The listing builds one solid part. Answer for the finished solid, in the listing's coordinates (mm). A direction names the side the tool comes from. Coordinates: 2 decimals unless noted, no trailing zeros. Order: outer loops, then holes, each group sorted by start corner. A loop starts at its lowest first (then second) coordinate and runs counter-clockwise, first axis right, second up. Notation, with made-up numbers: (83.5, -36.75) -> (99.5, -36.75) arc R13 cw to (99.5, -20.75) -> close; hole circle Ø4 at (9, 10). An arc over 180 degrees is marked (long way). Write each question's results on one line, items separated by ' | '. Start each with the question number.
(1) The part is cut by section B-B, the plane y = 13.25. Give the vertices of the cut face in (x, z).
(2) Straight lines are drawn through the part: L1, parallel to Y at x = 40, z = -40.5; L2, parallel to Z at x = -40.5, y = 14.5; L3, parallel to Z at x = -23.5, y = 1.5. For each, find the intervals that lie inside material, in ascending order.
(3) Determine the mould class of faces 3 (the face through (-50, 23, 24)), 4 (the face through (-53.3, 1, 14.7)), 5 (the face through (-0.195, -0.521, 61.487)), 6 (the face through (-62, 10.37, -19.52)) for opening direction Y: +Y half, -Y half, draft (parallel to the pull), parting line (faces both ways), or undercut.
(4) A tool of negligible diameter and unlimited length cuts with its end or side. For faces 1 (the face through (-53.3, 20, -14.7)), 2 (the face through (-0.195, 21.479, 61.487)), from which of +Z, -Z, +X, -X, +Y, -Y can it reach the whole face along a straight path? Write none if from no direction.
(5) The part is cut by section A-A, the plane z = -10. Give the vertices of the cut face in (x, y), then the cut area to 3 significant figures.
(6) The part is cut by section C-C, the plane x = -7.5. Give the vertices of the cut face in (y, z).
(7) Given pin 1 (2.5 mm diameter, centred on x = -51.96, z = 30, fed in from -Y); pin 2 (1.5 mm diameter, centred on x = -50, y = 2, fed in from +Z); pin 3 (8 mm diameter, centred on x = -29.5, y = 9.5, fed in from -Z); pin 4 (4 mm diameter, centred on y = 5, z = -50.5, fed in from +X), each flat-ended and moving along its own axis, determine where each tip first touches the part or whether it passes through.
Autodesk Inventor part; units mm, degrees
ref_plane "YZ Plane" through (0, 0, 0) normal (1, 0, 0) x (0, 1, 0)
ref_plane "XZ Plane" through (0, 0, 0) normal (0, 1, 0) x (-1, 0, 0)
ref_plane "XY Plane" through (0, 0, 0) normal (0, 0, 1) x (1, 0, 0)
sketch "Sketch1" plane through (0, 0, 0) normal (0, 1, 0) x (-1, 0, 0)
  circle A0 centre (0, 0) radius 65
  circle A1 centre (0, 0) radius 66.5
  dimension "d0" = 130
  dimension "d1" = 133
extrude "Extrusion1" add sketch "Sketch1" along normal blind 20
sketch "Sketch3" plane through (0, 0, 0) normal (0, -1, 0) x (1, 0, 0)
  circle A0 centre (0, -8) radius 1.5
  circle A1 centre (0, 8) radius 1.5
  circle A2 centre (9.5, 0) radius 1.5
  circle A3 centre (-9.5, 0) radius 1.5
  circle A4 centre (0, 0) radius 3.5464
  dimension "d11" = 3
  dimension "d12" = 8
  dimension "d13" = 3
  dimension "d14" = 9.5
extrude "Extrusion3" cut sketch "Sketch3" against normal blind 3
sketch "Sketch4" plane through (0, 0, 0) normal (0, -1, 0) x (1, 0, 0)
  circle A0 centre (0, 0) radius 66.5
  circle A1 centre (0, 0) radius 65
  dimension "d17" = 130
extrude "Extrusion4" add sketch "Sketch4" along normal blind 2
sketch "Sketch5" plane through (0, 20, 0) normal (0, 1, 0) x (1, 0, 0)
  circle A0 centre (0, 0) radius 66.5
  circle A1 centre (0, 0) radius 55
  dimension "d20" = 133
  dimension "d23" = 110
extrude "Extrusion5" add sketch "Sketch5" along normal blind 3
sketch "Sketch6" plane through (0, -2, 0) normal (0, -1, 0) x (1, 0, 0)
  circle A0 centre (0, 0) radius 66.5
  circle A1 centre (0, 0) radius 55
  dimension "d24" = 133
  dimension "d25" = 110
extrude "Extrusion6" add sketch "Sketch6" against normal blind 3
sketch "Sketch7" plane through (0, -2, 0) normal (0, -1, 0) x (1, 0, 0)
  circle A0 centre (0, -60) radius 1.5
  circle A1 centre (51.9615, -30) radius 1.5
  circle A2 centre (51.9615, 30) radius 1.5
  circle A3 centre (0, 60) radius 1.5
  circle A4 centre (-51.9615, 30) radius 1.5
  circle A5 centre (-51.9615, -30) radius 1.5
  point P0 (0, 0)
  dimension "d28" = 3
  dimension "d31" = 360
  dimension "d35" = 60
extrude "Extrusion7" cut sketch "Sketch7" against normal blind 1000
sketch "Sketch8" plane through (0, 23, 0) normal (0, 1, 0) x (1, 0, 0)
  circle A0 centre (0, 0) radius 55
  dimension "d36" = 110
properties part number "Motor mount (plain)"
Established:
1) outline: circle Ø133 at (0, 0); hole circle Ø130 at (0, 0)
2) L1: y = -2 to 1, 20 to 23 | L2: z = -52.74 to -50.84, 50.84 to 52.74 | L3: z = -62.21 to -60.6, 60.6 to 62.21
3) face 3: +Y half | face 4: undercut | face 5: draft | face 6: undercut
4) face 1: none | face 2: +Y, -Y
5) outline: (-65.74, -2) -> (-54.08, -2) -> (-54.08, 1) -> (-64.23, 1) -> (-64.23, 20) -> (-54.08, 20) -> (-54.08, 23) -> (-65.74, 23) -> close; (54.08, -2) -> (65.74, -2) -> (65.74, 23) -> (54.08, 23) -> (54.08, 20) -> (64.23, 20) -> (64.23, 1) -> (54.08, 1) -> close | area: 198 mm^2
6) outline: (-2, -66.08) -> (23, -66.08) -> (23, -54.49) -> (20, -54.49) -> (20, -64.57) -> (1, -64.57) -> (1, -54.49) -> (-2, -54.49) -> close; (-2, 54.49) -> (1, 54.49) -> (1, 64.57) -> (20, 64.57) -> (20, 54.49) -> (23, 54.49) -> (23, 66.08) -> (-2, 66.08) -> close
7) pin 1: passes through | pin 2: stops at z = 44.68 | pin 3: stops at z = -61.42 | pin 4: stops at x = 45.5
